CAD build for the part. Positions are in the model's coordinates, mm. A direction names the side the tool comes from. Round coordinates to 2 decimals unless told otherwise and drop trailing zeros. Write each loop counter-clockwise with the first axis right and the second up, starting at its lowest first coordinate (ties: lowest second). Pieces come first, ordered by that corner, then holes. Notation, with made-up numbers: (87, 32) - (94, 32) arc R17 cw to (94, 36) - close; hole circle Ø1 at (18, 54.5). An arc over 180 degrees is marked (long way). Put each result on its own line as item: value. Start each with the question number.
Item 1: 3-axis set-ups, long thin cutter, end or side, ignore diameter. For faces 5 (the flat face through (179.925, 1221.466, -124.93)), 6 (the cylindrical face through (153.204, 1248.243, -134.93)), 7 (the flat face through (175.5, 1172.9, -130)), 8 (the cylindrical face through (-23.295, 915.558, 4.93)), 9 (the flat face through (180.25, 1181.75, -124.93)): which of +Z, -Z, +X, -X, +Y, -Y reach the whole face in a straight line?
Item 2: Cut at A-A (z = -19.5). Give the cut face in (x, y), and give its area (3 significant figures).
Item 3: Mould opens along X. For faces 1 (the cylindrical face through (-28.164, 1139.625, 4.93)), 2 (the flat face through (361.15, 695.6, 4.93)), 3 (the cylindrical face through (398.94, 1252.49, 4.93)), 4 (the flat face through (345.016, 703.706, 4.93)) say: released by +X, released by -X, zero draft, split by the parting line, or undercut.
Item 4: Pin check, flat tips, straight feed: pin 1 Ø11 at (x, z) = (142.5, -123.5) entering from +Y; pin 2 Ø5 at (x, z) = (141, -83) entering from +Y; pin 3 Ø11 at (y, z) = (702, 6) entering from +X. Stop position of each tip, or through.
Item 5: Cut at C-C (y = 905.5). Give the cut face in (x, z), and give its area (3 significant figures).
Item 6: Cut at B-B (x = 223.5). Give the cut face in (y, z).
Item 7: Drill centre lines: line 1 (Z direction, x = 246, y = 468); line 2 (Z direction, x = 119, y = 1221); line 3 (Y direction, x = 136, z = -59.5). Where is each one in solid material? Low to high. Write a range as from..to.
```python
from build123d import *

# Parameters (mm, degrees)
BOSS_EXTRUDE1_DEPTH = 10
SKETCH3_W           = 9.565213244
SKETCH3_H           = 77.966410476
SKETCH3_W_2         = 8.353543979
SKETCH3_H_2         = 77.966410475
CUT_EXTRUDE1_DEPTH  = 250
SKETCH4_W           = 11
SKETCH4_H           = 97
CUT_EXTRUDE2_DEPTH  = 250
SKETCH5_R           = 25
BOSS_EXTRUDE2_DEPTH = 120
BOSS_EXTRUDE3_DEPTH = 10
SKETCH10_R          = 47.687508242
BOSS_EXTRUDE4_DEPTH = 10


with BuildPart() as part:
    # Sketch1 → Boss-Extrude1 (new body)
    with BuildSketch(Plane.XY):
        with BuildLine():
            Line((-51.984126252, 392.74957316), (0, 630.098149599))
            ThreePointArc((0, 630.098149599), (7.08288491, 733.363548715), (-3.984096645, 836.278231013))
            ThreePointArc((-3.984096645, 836.278231013), (-23.520457502, 916.694909006), (-36.012597338, 998.502353272))
            ThreePointArc((-36.012597338, 998.502353272), (-27.83897086, 1141.608720593), (10.535208392, 1279.716153066))
            ThreePointArc((10.535208392, 1279.716153066), (64.625002116, 1348.250843062), (147.435292888, 1375.912463775))
            ThreePointArc((147.435292888, 1375.912463775), (237.109169245, 1368.171524242), (318.838797646, 1330.467491469))
            ThreePointArc((318.838797646, 1330.467491469), (399.875156257, 1251.203752857), (450.033178317, 1149.548430819))
            ThreePointArc((450.033178317, 1149.548430819), (470.234397487, 1033.122029824), (450.033178317, 916.695628829))
            ThreePointArc((450.033178317, 916.695628829), (425.902967507, 824.914102712), (400.908098576, 733.364268538))
            ThreePointArc((400.908098576, 733.364268538), (374.881556851, 636.564375255), (358.063754215, 537.74756632))
            Line((358.063754215, 537.74756632), (308.99038073, 313.688874225))
            ThreePointArc((308.99038073, 313.688874225), (88.972777771, 172.731970202), (-51.984126252, 392.74957316))
        make_face()
    extrude(amount=BOSS_EXTRUDE1_DEPTH)

    # Sketch3 → Cut-Extrude1 (cut)
    with BuildSketch(Plane(origin=(0, 0, 0), x_dir=(-1, 0, 0), z_dir=(0, 0, -1))):
        with Locations((-4.782606622, 1061.735695438)):
            Rectangle(SKETCH3_W, SKETCH3_H)
        with Locations((11.17677199, 1061.735695438)):
            Rectangle(SKETCH3_W_2, SKETCH3_H)
        with Locations((-437.019311557, 1060.877248381)):
            Rectangle(SKETCH3_W_2, SKETCH3_H_2)
        with Locations((-421.059932945, 1060.448024852)):
            Rectangle(SKETCH3_W, SKETCH3_H_2)
    extrude(amount=-CUT_EXTRUDE1_DEPTH, mode=Mode.SUBTRACT)

    # Sketch4 → Cut-Extrude2 (cut)
    with BuildSketch(Plane(origin=(0, 0, 0), x_dir=(-1, 0, 0), z_dir=(0, 0, -1))):
        with Locations((-38.83297081, 691.059824561)):
            Rectangle(SKETCH4_W, SKETCH4_H)
        with Locations((-20.83297081, 691.059824561)):
            Rectangle(SKETCH4_W, SKETCH4_H)
        Polygon((-363.124216695, 747.966415693), (-326.394029606, 658.189506878), (-336.574916173, 654.024227929), (-373.305103262, 743.801136745), align=None)
        Polygon((-389.952232486, 736.954664741), (-353.222045397, 647.177755926), (-343.041158831, 651.343034874), (-379.77134592, 741.119943689), align=None)
    extrude(amount=-CUT_EXTRUDE2_DEPTH, mode=Mode.SUBTRACT)

    # Sketch5 → Boss-Extrude2 (add)
    with BuildSketch(Plane(origin=(0, 0, 0), x_dir=(-1, 0, 0), z_dir=(0, 0, -1))):
        with Locations(Location((-145.68729474, 1201.328438708, 0), (0, 0, 180))):
            Circle(SKETCH5_R)
    extrude(amount=BOSS_EXTRUDE2_DEPTH)

    # Sketch6 → Boss-Extrude3 (add)
    with BuildSketch(Plane(origin=(0, 0, -120), x_dir=(-1, 0, 0), z_dir=(0, 0, -1))):
        Polygon((-99.823082616, 1201.328438708), (-122.755188678, 1241.048011532), (-168.619400802, 1241.048011532), (-191.551506864, 1201.328438708), (-168.619400802, 1161.608865884), (-122.755188678, 1161.608865884), align=None)
    extrude(amount=BOSS_EXTRUDE3_DEPTH)

    # Sketch10 → Boss-Extrude4 (add)
    with BuildSketch(Plane(origin=(0, 0, -130), x_dir=(-1, 0, 0), z_dir=(0, 0, -1))):
        with Locations((-146.996021508, 1200.961482621)):
            Circle(SKETCH10_R)
    extrude(amount=BOSS_EXTRUDE4_DEPTH)


solid = part.part
```
Output values:
1. face 5: +X, +Y
1. face 6: -Z
1. face 7: none
1. face 8: +Z, -Z, -X
1. face 9: +X, -Y
2. outline: circle Ø50 at (145.69, 1201.33)
2. area: 1,960 mm2
3. face 1: released by -X
3. face 2: undercut
3. face 3: released by +X
3. face 4: undercut
4. pin 1: y = 1241.05
4. pin 2: y = 1226.23
4. pin 3: x = 392.99
5. outline: (-21.24, 0) - (447.14, 0) - (447.14, 10) - (-21.24, 10) - close
5. area: 4,680 mm2
6. outline: (194.75, 0) - (1371.39, 0) - (1371.39, 10) - (194.75, 10) - close
7. line 1: 0..10
7. line 2: -140..-120, 0..10
7. line 3: 1178.28..1224.38
